```python
from build123d import *

# Parameters (mm, degrees)
SKETCH_1_W          = 229
SKETCH_1_H          = 79.5
EXTRUDE_1_DEPTH     = 10
FILLET_1_R          = 10
SKETCH_2_R          = 2.1
CUT_EXTRUDE_1_DEPTH = 122.615428709
CUT_EXTRUDE_2_DEPTH = 4.5
CUT_EXTRUDE_3_DEPTH = 122.615428709
FILLET_2_R          = 4
CUT_EXTRUDE_4_DEPTH = 122.615428709
FILLET_3_R          = 2


with BuildPart() as part:
    # 草图1 → 凸台-拉伸1 (new body)
    with BuildSketch(Plane.XY):
        Rectangle(SKETCH_1_W, SKETCH_1_H)
    extrude(amount=EXTRUDE_1_DEPTH)

    # 圆角1
    fillet_1_edges = [part.edges().sort_by_distance(p)[0] for p in [
        (114.5, -39.75, 5),
        (-114.5, -39.75, 5),
        (-114.5, 39.75, 5),
        (114.5, 39.75, 5),
    ]]
    fillet(fillet_1_edges, radius=FILLET_1_R)

    # 草图2 → 切除-拉伸1 (cut, through all)
    with BuildSketch(Plane(origin=(0, 0, 0), x_dir=(-1, 0, 0), z_dir=(0, 0, -1))):
        with Locations((99.5, 25)):
            Circle(SKETCH_2_R)
        with Locations(Location((99.5, -25, 0), (0, 0, 180))):
            Circle(SKETCH_2_R)
        with Locations((-99.5, -25)):
            Circle(SKETCH_2_R)
        with Locations(Location((-99.5, 25, 0), (0, 0, 180))):
            Circle(SKETCH_2_R)
    extrude(amount=-CUT_EXTRUDE_1_DEPTH, mode=Mode.SUBTRACT)

    # 草图3 → 切除-拉伸2 (cut)
    with BuildSketch(Plane(origin=(0, 0, 0), x_dir=(-1, 0, 0), z_dir=(0, 0, -1))):
        Polygon((-97.392671517, 21.35), (-95.285343035, 25), (-97.392671517, 28.65), (-101.607328483, 28.65), (-103.714656965, 25), (-101.607328483, 21.35), align=None)
        Polygon((-97.392671517, -28.65), (-95.285343035, -25), (-97.392671517, -21.35), (-101.607328483, -21.35), (-103.714656965, -25), (-101.607328483, -28.65), align=None)
        Polygon((101.607328483, 21.35), (103.714656965, 25), (101.607328483, 28.65), (97.392671517, 28.65), (95.285343035, 25), (97.392671517, 21.35), align=None)
        Polygon((101.607328483, -28.65), (103.714656965, -25), (101.607328483, -21.35), (97.392671517, -21.35), (95.285343035, -25), (97.392671517, -28.65), align=None)
    extrude(amount=-CUT_EXTRUDE_2_DEPTH, mode=Mode.SUBTRACT)

    # 草图4 → 切除-拉伸3 (cut, through all)
    with BuildSketch(Plane(origin=(0, 0, 0), x_dir=(-1, 0, 0), z_dir=(0, 0, -1))):
        Polygon((-80, 39.75), (-34.966679003, 13.75), (34.966679003, 13.75), (80, 39.75), align=None)
        Polygon((80, -39.75), (34.966679003, -13.75), (-34.966679003, -13.75), (-80, -39.75), align=None)
    extrude(amount=-CUT_EXTRUDE_3_DEPTH, mode=Mode.SUBTRACT)

    # 圆角2
    fillet_2_edges = [part.edges().sort_by_distance(p)[0] for p in [
        (80, 39.75, 5),
        (-80, 39.75, 5),
        (-34.966679003, 13.75, 5),
        (34.966679003, 13.75, 5),
        (-80, -39.75, 5),
        (80, -39.75, 5),
        (34.966679003, -13.75, 5),
        (-34.966679003, -13.75, 5),
    ]]
    fillet(fillet_2_edges, radius=FILLET_2_R)

    # 草图6 → 切除-拉伸4 (cut, through all)
    with BuildSketch(Plane(origin=(0, 0, 0), x_dir=(-1, 0, 0), z_dir=(0, 0, -1))):
        Polygon((-82.657935628, 35.511057159), (-94.5, 15), (-94.5, 5), (-4, 5), (-4, 8.75), (-36.306424965, 8.75), align=None)
        Polygon((36.306424965, 8.75), (82.657935628, 35.511057159), (94.5, 15), (94.5, 5), (4, 5), (4, 8.75), align=None)
        Polygon((82.657935628, -35.511057159), (94.5, -15), (94.5, -5), (4, -5), (4, -8.75), (36.306424965, -8.75), align=None)
        Polygon((-36.306424965, -8.75), (-82.657935628, -35.511057159), (-94.5, -15), (-94.5, -5), (-4, -5), (-4, -8.75), align=None)
    extrude(amount=-CUT_EXTRUDE_4_DEPTH, mode=Mode.SUBTRACT)

    # 圆角3
    # the kernel refuses this fillet: 2 mm, written as the material it adds along each edge
    with BuildSketch(Plane(origin=(4, 8.75, 0), x_dir=(0, -1, 0), z_dir=(0, 0, 1)), Plane(origin=(94.5, 5, 0), x_dir=(0, 1, 0), z_dir=(0, 0, 1)), Plane(origin=(4, 5, 0), x_dir=(1, 0, 0), z_dir=(0, 0, 1)), Plane(origin=(-82.657935628, 35.511057159, 0), x_dir=(-0.499999999999999, -0.8660254037844393, 0), z_dir=(0, 0, 1)), Plane(origin=(-4, 5, 0), x_dir=(0, 1, 0), z_dir=(0, 0, 1)), Plane(origin=(-4, 8.75, 0), x_dir=(-1, 0, 0), z_dir=(0, 0, 1)), Plane(origin=(-94.5, 5, 0), x_dir=(1, 0, 0), z_dir=(0, 0, 1)), Plane(origin=(82.657935628, -35.511057159, 0), x_dir=(0.5000000000000006, 0.8660254037844384, 0), z_dir=(0, 0, 1)), Plane(origin=(94.5, -5, 0), x_dir=(-1, 0, 0), z_dir=(0, 0, 1)), Plane(origin=(4, -5, 0), x_dir=(0, -1, 0), z_dir=(0, 0, 1)), Plane(origin=(4, -8.75, 0), x_dir=(1, 0, 0), z_dir=(0, 0, 1)), Plane(origin=(-4, -8.75, 0), x_dir=(0, 1, 0), z_dir=(0, 0, 1)), Plane(origin=(-4, -5, 0), x_dir=(-1, 0, 0), z_dir=(0, 0, 1)), Plane(origin=(-94.5, -5, 0), x_dir=(0, -1, 0), z_dir=(0, 0, 1))) as fillet_3_piece_1:
        with BuildLine():
            CenterArc((FILLET_3_R, FILLET_3_R), FILLET_3_R, 180, 90)
            Line((0, FILLET_3_R), (0, 0))
            Line((0, 0), (FILLET_3_R, 0))
        make_face()
    extrude(amount=10)
    with BuildSketch(Plane(origin=(94.5, 15, 0), x_dir=(-0.5000000000000042, 0.8660254037844363, 0), z_dir=(0, 0, 1)), Plane(origin=(-94.5, 15, 0), x_dir=(0, -1, 0), z_dir=(0, 0, 1)), Plane(origin=(94.5, -15, 0), x_dir=(0, 1, 0), z_dir=(0, 0, 1)), Plane(origin=(-94.5, -15, 0), x_dir=(0.49999999999999856, -0.8660254037844396, 0), z_dir=(0, 0, 1))) as fillet_3_piece_2:
        with BuildLine():
            CenterArc((FILLET_3_R * 0.267949192431, FILLET_3_R), FILLET_3_R, 240, 30)
            Line((-FILLET_3_R * 0.232050807569, FILLET_3_R * 0.133974596216), (0, 0))
            Line((0, 0), (FILLET_3_R * 0.267949192431, 0))
        make_face()
    extrude(amount=10)
    with BuildSketch(Plane(origin=(82.657935628, 35.511057159, 0), x_dir=(0.499999999999999, -0.8660254037844393, 0), z_dir=(0, 0, 1)), Plane(origin=(-82.657935628, -35.511057159, 0), x_dir=(-0.499999999999999, 0.8660254037844393, 0), z_dir=(0, 0, 1))) as fillet_3_piece_3:
        with BuildLine():
            CenterArc((FILLET_3_R, -FILLET_3_R), FILLET_3_R, 90, 90)
            Line((0, -FILLET_3_R), (0, 0))
            Line((0, 0), (FILLET_3_R, 0))
        make_face()
    extrude(amount=10)
    # the kernel refuses this fillet: 2 mm, written as the material it takes off along each edge
    with BuildSketch(Plane(origin=(36.306424965, 8.75, -1.339745962), x_dir=(-1, 0, 0), z_dir=(0, 0, 1)), Plane(origin=(-36.306424965, -8.75, -1.339745962), x_dir=(1, 0, 0), z_dir=(0, 0, 1))) as fillet_3_2_piece_1:
        with BuildLine():
            CenterArc((FILLET_3_R * 0.267949192431, -FILLET_3_R), FILLET_3_R, 90, 30)
            Line((-FILLET_3_R * 0.232050807569, -FILLET_3_R * 0.133974596216), (0, 0))
            Line((0, 0), (FILLET_3_R * 0.267949192431, 0))
        make_face()
    extrude(amount=12.679491924, mode=Mode.SUBTRACT)
    with BuildSketch(Plane(origin=(-36.306424965, 8.75, -1.339745962), x_dir=(1, 0, 0), z_dir=(0, 0, 1)), Plane(origin=(36.306424965, -8.75, -1.339745962), x_dir=(-1, 0, 0), z_dir=(0, 0, 1))) as fillet_3_2_piece_2:
        with BuildLine():
            CenterArc((FILLET_3_R * 0.267949192431, FILLET_3_R), FILLET_3_R, 240, 30)
            Line((-FILLET_3_R * 0.232050807569, FILLET_3_R * 0.133974596216), (0, 0))
            Line((0, 0), (FILLET_3_R * 0.267949192431, 0))
        make_face()
    extrude(amount=12.679491924, mode=Mode.SUBTRACT)


solid = part.part
```
The listing builds one solid part. Answer for the finished solid, in the listing's coordinates (mm). A direction names the side the tool comes from. Give positions to 0.01 mm unless a question says otherwise; leave off trailing zeros. Order: outer loops, then holes, each group sorted by start corner. A loop starts at its lowest first (then second) coordinate and runs counter-clockwise, first axis right, second up. Notation, with made-up numbers: (1, 0.25) - (12, 0.25) arc R9 cw to (12, 5.25) - close; hole circle Ø4 at (-14, -15). An arc over 180 degrees is marked (long way). Answer in a Markdown table with one row per item. Add a question column.
Q1. For a pull along Y with two mould halves and no side action, classify faces 1 (the flat face through (0, -13.75, 5)), 2 (the flat face through (114.5, 0, 5)), 3 (the flat face through (102.676, -26.799, 2.218)) as released by +Y, released by -Y, zero draft, split by the parting line, or undercut.
Q2. The part is cut by section D-D (x = 99.5). Determine the outline of the cut face in (y, z).
Q3. The part is cut by section A-A (x = 17). Determine the outline of the cut face in (y, z), then the cut area to 3 significant figures.
Q4. Which of the six approach directions +Z, -Z, +X, -X, +Y, -Y give full straight-line access (tool end or side, diameter ignored) to faces 4 (the flat face through (-57.786, -26.924, 4.93)), 5 (the flat face through (102.646, -23.149, 2.218)), 6 (the flat face through (58.539, 21.586, 4.93))?
Q5. Find the intervals of material crossed by line 1 along Y through (x, z) = (97.5, 1.25); line 2 along Y through (x, z) = (-15.5, 7.75); line 3 along X through (y, z) = (-12.5, 5.75), in increasing order. Write a range as [from, to].
Q6. The part is cut by section C-C (z = 8). Give the number of separate pieces and of enclosed holes in the cut face, then the cut area to 3 significant figures.
Q7. The part is cut by section B-B (y = -18). Determine the outline of the cut face in (x, z), then the cut area to 3 significant figures.
Q8. Given P1, Ø3, axis at x = -46, z = 6, coming from the -Y side; P2, Ø5, axis at x = 15.5, z = 3.5, coming from the +Y side, each flat-ended and moving along its own axis, determine where each tip first touches the part or whether it passes through.
Determined:
| question | item | result |
|---|---|---|
| 1 | face 1 | released by -Y |
| 1 | face 2 | zero draft |
| 1 | face 3 | undercut |
| 2 | outline | (-39.75, 0) - (-28.65, 0) - (-28.65, 4.5) - (-27.1, 4.5) - (-27.1, 10) - (-39.75, 10) - close; (-22.9, 4.5) - (-21.35, 4.5) - (-21.35, 0) - (21.35, 0) - (21.35, 4.5) - (22.9, 4.5) - (22.9, 10) - (-22.9, 10) - close; (27.1, 4.5) - (28.65, 4.5) - (28.65, 0) - (39.75, 0) - (39.75, 10) - (27.1, 10) - close |
| 3 | outline | (-13.75, 0) - (-8.75, 0) - (-8.75, 10) - (-13.75, 10) - close; (-5, 0) - (5, 0) - (5, 10) - (-5, 10) - close; (8.75, 0) - (13.75, 0) - (13.75, 10) - (8.75, 10) - close |
| 3 | area | 200 mm² |
| 4 | face 4 | +Z, -Z, -Y |
| 4 | face 5 | -Z |
| 4 | face 6 | +Z, -Z |
| 5 | line 1 | y = [-39.75, -28.65], [-21.35, 21.35], [28.65, 39.75] |
| 5 | line 2 | y = [-13.75, -8.75], [-5, 5], [8.75, 13.75] |
| 5 | line 3 | x = [-114.5, -94.5], [-42.8, 42.8], [94.5, 114.5] |
| 6 | separate pieces | 1 |
| 6 | enclosed holes | 8 |
| 6 | area | 7,480 mm² |
| 7 | outline | (-114.5, 0) - (-92.77, 0) - (-92.77, 10) - (-114.5, 10) - close; (-52.33, 0) - (-42.33, 0) - (-42.33, 10) - (-52.33, 10) - close; (42.33, 0) - (52.33, 0) - (52.33, 10) - (42.33, 10) - close; (92.77, 0) - (114.5, 0) - (114.5, 10) - (92.77, 10) - close |
| 7 | area | 635 mm² |
| 8 | P1 | stops at y = -20.99 |
| 8 | P2 | stops at y = 13.75 |
